```python
from build123d import *

# Parameters (mm, degrees)
BOSS_EXTRUDE1_DEPTH      = 15.24
BOSS_EXTRUDE1_DEPTH_BACK = 76.2
FILLET1_R                = 1.27
BOSS_EXTRUDE2_DEPTH      = 8.04
CUT_EXTRUDE1_DEPTH       = 50.8
CUT_EXTRUDE2_DEPTH       = 38.1
CUT_EXTRUDE3_DEPTH       = 38.1


with BuildPart() as part:
    # Sketch3 → Boss-Extrude1 (new, two sides: drawn at the far end of the back side and taken through both)
    with BuildSketch(Plane(origin=(0, 0, 0), x_dir=(1, 0, 0), z_dir=(0, 1, 0)).offset(-BOSS_EXTRUDE1_DEPTH_BACK)):
        with BuildLine():
            Line((-475.15475454, -2.10083146), (-513.153172489, -2.10083146))
            Line((-513.153172489, -2.10083146), (-539.064824243, -44.116848998))
            Line((-539.064824243, -44.116848998), (-532.913087574, -96.64839438))
            ThreePointArc((-532.913087574, -96.64839438), (-438.150016702, -46.02), (-343.386945829, -96.64839438))
            Line((-343.386945829, -96.64839438), (-349.858652302, -50.677017736))
            Line((-349.858652302, -50.677017736), (-383.060284532, -2.10083146))
            Line((-383.060284532, -2.10083146), (-449.75475454, -2.10083146))
            ThreePointArc((-449.75475454, -2.10083146), (-462.45475454, -14.80083146), (-475.15475454, -2.10083146))
        make_face()
    extrude(amount=BOSS_EXTRUDE1_DEPTH + BOSS_EXTRUDE1_DEPTH_BACK)

    # Fillet1
    fillet1_edges = [part.edges().sort_by_distance(p)[0] for p in [
        (-532.913087574, -30.48, 96.64839438),
        (-343.386945829, -30.48, 96.64839438),
    ]]
    fillet(fillet1_edges, radius=FILLET1_R)

    # Sketch4 → Boss-Extrude2 (add)
    with BuildSketch(Plane(origin=(0, 15.24, 0), x_dir=(1, 0, 0), z_dir=(0, 1, 0))):
        with BuildLine():
            Line((-380.135465932, -93.16197835), (-345.369151466, -92.873286736))
            ThreePointArc((-345.369151466, -92.873286736), (-439.104227144, -45.107135711), (-532.033153207, -94.423302399))
            Line((-532.033153207, -94.423302399), (-497.266838741, -94.134610785))
            ThreePointArc((-497.266838741, -94.134610785), (-438.886956078, -71.272475515), (-380.135465932, -93.16197835))
        make_face()
    extrude(amount=-BOSS_EXTRUDE2_DEPTH)

    # Sketch5 → Cut-Extrude1 (cut)
    with BuildSketch(Plane(origin=(0, 15.24, 0), x_dir=(1, 0, 0), z_dir=(0, 1, 0))):
        with BuildLine():
            Line((-528.314052027, -40.689759741), (-516.187462201, -44.462798197))
            Line((-516.187462201, -44.462798197), (-527.50657757, -80.842567675))
            Line((-527.50657757, -80.842567675), (-695.232596141, -28.656691245))
            ThreePointArc((-695.232596141, -28.656691245), (-715.264918055, 13.486917548), (-671.654107709, 30.084354228))
            ThreePointArc((-671.654107709, 30.084354228), (-668.860719824, 16.856608708), (-682.026961544, 13.786373146))
            ThreePointArc((-682.026961544, 13.786373146), (-697.926589826, 5.432821776), (-689.573038456, -10.466806506))
            Line((-689.573038456, -10.466806506), (-533.973609712, -58.87964448))
            Line((-533.973609712, -58.87964448), (-528.314052027, -40.689759741))
        make_face()
    extrude(amount=-CUT_EXTRUDE1_DEPTH, mode=Mode.SUBTRACT)

    # Sketch6 → Cut-Extrude2 (cut)
    with BuildSketch(Plane(origin=(0, 15.24, 0), x_dir=(1, 0, 0), z_dir=(0, 1, 0))):
        Polygon((-505.199519379, -28.941561379), (-510.924193781, -42.454904444), (-475.918740123, -42.454904444), (-475.918740123, -28.941649602), align=None)
    extrude(amount=-CUT_EXTRUDE2_DEPTH, mode=Mode.SUBTRACT)

    # Sketch7 → Cut-Extrude3 (cut)
    with BuildSketch(Plane.XZ.offset(76.2)):
        with BuildLine():
            Line((-477.784341144, 30.750375257), (-493.297876549, 29.59254273))
            ThreePointArc((-493.297876549, 29.59254273), (-509.568926068, 36.66140776), (-512.958981795, 54.074719549))
            Line((-512.958981795, 54.074719549), (-477.784341144, 43.499133869))
            Line((-477.784341144, 43.499133869), (-477.784341144, 30.750375257))
        make_face()
    extrude(amount=-CUT_EXTRUDE3_DEPTH, mode=Mode.SUBTRACT)


solid = part.part
```
Source: CAD feature listing. Evaluate the final solid. Frame: model axes, mm. A direction names the side the tool comes from. Give positions to 0.01 mm unless a question says otherwise; leave off trailing zeros. Loops run counter-clockwise (first coordinate to the right, second up) from the corner with the lowest first, then second, coordinate; pieces in that order, holes last. Notation, with made-up numbers: (-35, 66) -> (-2, 66) arc R18 cw to (-2, 85) -> close; hole circle Ø8 at (38, 68). An arc over 180 degrees is marked (long way). Put each result on its own line as item: value. Start each with the question number.
1) Draft query along X for faces 1 (the face through (-494, -4, 42.455)), 2 (the face through (-416, -31, 2.101)), 3 (the face through (-366.227, -31.12, 26.729)), 4 (the face through (-496, -38.1, 39)). Return one class per face: released by +X, released by -X, zero draft, split by the parting line, or undercut.
2) Material intervals for probe 1 along Y at (x, z) = (-496.5, 47); probe 2 along X at (y, z) = (-9.5, 77); probe 3 along X at (y, z) = (-36, 72), sorted ascending.
3) Cut plane B-B (y = -49). Return loops of the section in (x, z), then the cut area to 3 significant figures.
4) Contact query for flat-ended pins moving along their axis: P1, Ø3, axis at y = -53, z = 77, coming from the +X side; P2, Ø10, axis at y = -4, z = 12.5, coming from the -X side; P3, Ø7, axis at x = -488.5, z = 33, coming from the +Y side; P4, Ø23.5, axis at x = -531.5, z = 56.5, coming from the +Y side. Output: stop coordinate, or through.
5) Cut plane D-D (z = 74). Return loops of the section in (x, y).
6) Cut plane C-C (x = -523.5). Return loops of the section in (y, z), then the cut area to 3 significant figures.
7) Reachability of faces 5 (the face through (-443, -76.2, 37)), 6 (the face through (-522.34, -9.8, 42.55)), 7 (the face through (-509.406, -57.417, 36.461)), 8 (the face through (-440, 7.2, 70)) from +Z, -Z, +X, -X, +Y, -Y: full face, straight path, thin tool, end or side. Return the list, or none.
8) Cut plane A-A (z = 84.5). Return loops of the section in (x, y), then the cut area to 3 significant figures.
Results are:
1. face 1: undercut
1. face 2: zero draft
1. face 3: released by +X
1. face 4: undercut
2. probe 1: y = -38.1 to 15.24
2. probe 2: x = -526.31 to -516.28, -360.02 to -346.15
2. probe 3: x = -535.8 to -510.6, -365.7 to -346.86
3. outline: (-539.06, 44.12) -> (-513.15, 2.1) -> (-475.15, 2.1) arc R12.7 cw to (-449.75, 2.1) -> (-383.06, 2.1) -> (-349.86, 50.68) -> (-344.12, 91.43) arc R1.27 ccw to (-346.4, 92.36) arc R114 cw to (-531.01, 93.89) arc R1.27 ccw to (-533.31, 93.3) -> close; hole (-512.96, 54.07) arc R19.05 ccw to (-493.3, 29.59) -> (-477.78, 30.75) -> (-477.78, 43.5) -> close
3. area: 8,910 mm2
4. P1: stops at x = -345.94
4. P2: stops at x = -522.65
4. P3: stops at y = -22.86
4. P4: stops at y = 15.24
5. outline: (-535.57, -76.2) -> (-512.96, -76.2) -> (-512.96, 7.2) -> (-459.89, 7.2) -> (-459.89, 15.24) -> (-525.38, 15.24) -> (-525.38, -35.56) -> (-535.57, -35.56) -> close; (-416.43, 7.2) -> (-363.34, 7.2) -> (-363.34, -76.2) -> (-346.58, -76.2) -> (-346.58, 15.24) -> (-416.43, 15.24) -> close
6. outline: (-76.2, 18.88) -> (15.24, 18.88) -> (15.24, 42.19) -> (-35.56, 42.19) -> (-35.56, 67.97) -> (15.24, 67.97) -> (15.24, 94.35) -> (7.2, 94.35) -> (7.2, 84.45) -> (-76.2, 84.45) -> close
6. area: 4,770 mm2
7. face 5: +Z, -Z, +X, -X, -Y
7. face 6: +Y
7. face 7: -Y
7. face 8: +Z, -Y
8. outline: (-534.34, -76.2) -> (-523.55, -76.2) -> (-523.55, 7.2) -> (-484.52, 7.2) -> (-484.52, 15.24) -> (-534.34, 15.24) -> close; (-391.8, 7.2) -> (-352.75, 7.2) -> (-352.75, -76.2) -> (-345.1, -76.2) -> (-345.1, 15.24) -> (-391.8, 15.24) -> close
8. area: 2,310 mm2
